Geometry: see drawing. Coordinates: mm, zero at the bounding-box minimum. A direction names the side the tool comes from. Give positions to 0.01 mm unless a question says otherwise; leave off trailing zeros. Write each loop counter-clockwise with the first axis right and the second up, starting at its lowest first coordinate (ties: lowest second). Pieces come first, ordered by that corner, then holes. Notation, with made-up numbers: (17.5, 89.5) -> (63.5, 89.5) arc R12 cw to (63.5, 105.5) -> close; hole circle Ø9 at (51.25, 42). An arc over 180 degrees is marked (long way). Use one line per item in the form item = value. Start each with the question number.
(1) Cut plane D-D, the plane z = 5. Output: boundary loops of the cut face in (x, y).
(2) Cut plane B-B, the plane y = 1.5. Output: boundary loops of the cut face in (x, z), and give its area (3 significant figures).
(3) First-contact query: P1, Ø3, axis at y = 8, z = 33, coming from the -X side; P2, Ø1.6, axis at x = 19, y = 11, coming from the -Z side; P3, Ø1.5, axis at x = 5.5, y = 1.5, coming from the +Z side; P4, Ø2.5, axis at x = 25, z = 20, coming from the -Y side. Flat tips, straight axial feed; report the tip coordinate or a pass-through.
(4) Cut plane C-C, the plane x = 6. Output: boundary loops of the cut face in (y, z).
(5) Draft query along Z for the marked faces 1, 2 and 3. Return one class per face: pulls with the +Z half, pulls with the -Z half, needs draft (parallel to the pull), parting line crosses it, or undercut.
(6) Set-up query: the marked faces 4, 5 and 6. Return all of +Z, -Z, +X, -X, +Y, -Y with unobstructed straight access to the full face (end or side cutting, diameter ignored); none if empty.
(7) Material intervals for line 1 along Z through (x, y) = (10, 5.75); line 2 along Y through (x, z) = (33.5, 19); line 3 along Y through (x, z) = (36, 34), sorted ascending. Write a range as from..to.
(8) Cut plane A-A, the plane x = 10. Output: boundary loops of the cut face in (y, z).
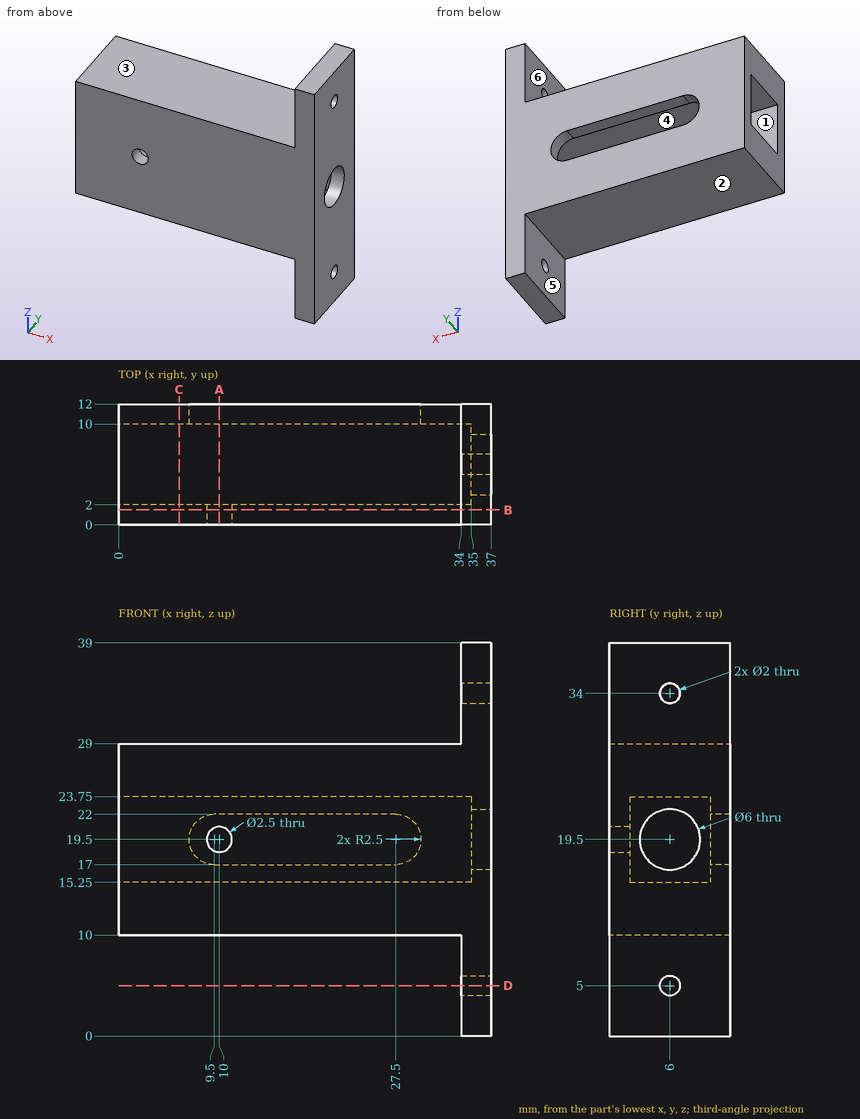
Geometry says:
q1.outline = (34, 0) -> (37, 0) -> (37, 5) -> (34, 5) -> close; (34, 7) -> (37, 7) -> (37, 12) -> (34, 12) -> close
q2.outline = (0, 10) -> (34, 10) -> (34, 0) -> (37, 0) -> (37, 39) -> (34, 39) -> (34, 29) -> (0, 29) -> close; hole circle Ø2.5 at (10, 19.5)
q2.area = 758 mm^2
q3.P1 = 34
q3.P2 = 10
q3.P3 = 29
q3.P4 = 0
q4.outline = (0, 10) -> (12, 10) -> (12, 29) -> (0, 29) -> close; hole (2, 15.25) -> (10, 15.25) -> (10, 23.75) -> (2, 23.75) -> close
q5.face_1 = undercut
q5.face_2 = pulls with the -Z half
q5.face_3 = pulls with the +Z half
q6.face_4 = -X
q6.face_5 = -Z, -X, +Y, -Y
q6.face_6 = +Z, -X, +Y, -Y
q7.line_1 = 10..15.25, 23.75..29
q7.line_2 = 0..2, 10..12
q7.line_3 = 0..5, 7..12
q8.outline = (0, 10) -> (12, 10) -> (12, 17) -> (10, 17) -> (10, 15.25) -> (2, 15.25) -> (2, 18.25) -> (0, 18.25) -> close; (0, 20.75) -> (2, 20.75) -> (2, 23.75) -> (10, 23.75) -> (10, 22) -> (12, 22) -> (12, 29) -> (0, 29) -> close
